Autodesk Inventor part; units mm, degrees
ref_plane "YZ Plane" through (0, 0, 0) normal (1, 0, 0) x (0, 1, 0)
ref_plane "XZ Plane" through (0, 0, 0) normal (0, 1, 0) x (-1, 0, 0)
ref_plane "XY Plane" through (0, 0, 0) normal (0, 0, 1) x (1, 0, 0)
sketch "Sketch1" plane through (0, 0, 0) normal (0, 0, 1) x (1, 0, 0)
  circle A0 centre (0, 0) radius 8
  line L0 (0, 0) -> (-8.735, 0) construction
  line L1 (0, 0) -> (-17.865, 0) construction
  line L2 (-8.735, 0) -> (-8.735, 11) construction
  line L3 (-8.735, 0) -> (-8.735, -11) construction
  line L4 (-17.865, 0) -> (-17.865, -11) construction
  line L5 (-17.865, 0) -> (-17.865, 11) construction
  line L6 (8, 0) -> (15, 0) construction
  line L7 (-17.865, 0) -> (-22.365, 0) construction
  line L8 (-22.365, -11) -> (15, -11)
  line L9 (15, -11) -> (15, 11)
  line L10 (15, 11) -> (-22.365, 11)
  line L11 (-22.365, 11) -> (-22.365, -11)
  dimension "d0" = 16
  dimension "d1" = 8.735
  dimension "d2" = 17.865
  dimension "d3" = 11
  dimension "d4" = 11
  dimension "d5" = 11
  dimension "d6" = 11
  dimension "d7" = 7
  dimension "d8" = 4.5
  dimension "d23" = 37.365
extrude "Extrusion1" add sketch "Sketch1" along normal mid plane 11
sketch "Sketch2" plane through (-22.365, 11, 5.5) normal (0, 1, 0) x (1, 0, 0)
  line L0 (0, 11) -> (0, 0)
  line L1 (0, 5.5) -> (4.5, 5.5)
  line L2 (4.5, 5.5) -> (13.63, 5.5)
  circle A0 centre (4.5, 5.5) radius 1.5
  circle A1 centre (13.63, 5.5) radius 1.75
  point P0 (22.365, 5.5)
  dimension "d11" = 4.5
  dimension "d13" = 9.13
  dimension "d14" = 3
  dimension "d15" = 3.5
extrude "Extrusion2" cut sketch "Sketch2" against normal up to next contours A0 L2 L1 | L1 L2 A0
extrude "Extrusion3" cut sketch "Sketch2" against normal blind 4 contours A1
sketch "Sketch3" plane through (-22.365, -11, 5.5) normal (0, -1, 0) x (1, 0, 0)
  circle A0 centre (13.63, -5.5) radius 1.75
  circle A1 centre (13.63, -5.5) radius 1.75
  point P0 (22.365, -5.5)
extrude "Extrusion4" cut sketch "Sketch3" against normal blind 4
fillet "Fillet1" radius 5.5 4 edges at (-22.365, 0, 5.5) (15, 0, 5.5) (15, 0, -5.5) (-22.365, 0, -5.5)
equation "\"d23\" = d2 + d7 + 0.5 * d0 + d8"
properties part number "ArmMidClip - 16mmBore"
Here's how the part is built. I have some questions about the finished solid (model axes, mm). A direction names the side the tool comes from. Round coordinates to 2 decimals unless told otherwise and drop trailing zeros. Write each loop counter-clockwise with the first axis right and the second up, starting at its lowest first coordinate (ties: lowest second). Pieces come first, ordered by that corner, then holes.
Q1. If we section it at B-B on y = 0: Give the number of separate pieces and of enclosed holes in the cut face, plus the area to 3 significant figures.
Q2. If we mould it in two halves opening along X, with no side actions, what happens to faces 1 (the cylindrical face through (13.43, 0.15, -3.85)), 2 (the cylindrical face through (-19.364, 0.154, -0.066)), 3 (the flat face through (-3, 11, 0))? For each: +X half, -X half, draft (parallel to the pull), parting line (faces both ways), or undercut.
Q3. Which directions (+Z, -Z, +X, -X, +Y, -Y) give clear straight access to the entire face, cutting with the end or side of a thin tool? Please do faces 4 (the cylindrical face through (-10.483, -9.028, 0.077)), 5 (the cylindrical face through (-20.711, -0.154, 3.932)), 6 (the flat face through (-9, 7, 0)).
Q4. Please list where these lines run through material, in increasing order: probe 1 along Y at (x, z) = (0, -3.5); probe 2 along X at (y, z) = (-2.5, 1); probe 3 along X at (y, z) = (4, 0) (3 decimals).
Q5. If we section it at C-C on x = -7.5: Write out the boundary of the cut face in (y, z).
Q6. If we section it at A-A on x = 0: Write out the boundary of the cut face in (y, z).
Q7. Will these pins go through, and if not, where does the flat tip stop? P1, Ø1, axis at x = -8.5, z = 0.5, coming from the -Y side; P2, Ø1, axis at y = -6, z = -1.5, coming from the +X side; P3, Ø1, axis at y = -7, z = 3, coming from the -X side; P4, Ø1.8, axis at x = -17.865, z = 0, coming from the +Y side.
Answer below:
1. separate pieces: 2
1. enclosed holes: 1
1. area: 202 mm2
2. face 1: +X half
2. face 2: undercut
2. face 3: draft
3. face 4: -Y
3. face 5: +Z, -X, +Y, -Y
3. face 6: +Y
4. probe 1: y = -11 to -8, 8 to 11
4. probe 2: x = -22.27 to -18.98, -16.75 to -7.6, 7.6 to 14.91
4. probe 3: x = -22.365 to -19.365, -16.365 to -6.928, 6.928 to 15
5. outline: (-11, -5.5) - (-2.78, -5.5) - (-2.78, 5.5) - (-11, 5.5) - (-11, 1.24) - (-7, 1.24) - (-7, -1.24) - (-11, -1.24) - close; (2.78, -5.5) - (11, -5.5) - (11, -1.24) - (7, -1.24) - (7, 1.24) - (11, 1.24) - (11, 5.5) - (2.78, 5.5) - close
6. outline: (-11, -5.5) - (-8, -5.5) - (-8, 5.5) - (-11, 5.5) - close; (8, -5.5) - (11, -5.5) - (11, 5.5) - (8, 5.5) - close
7. P1: stops at y = -7
7. P2: stops at x = 14.91
7. P3: stops at x = -21.76
7. P4: passes through
